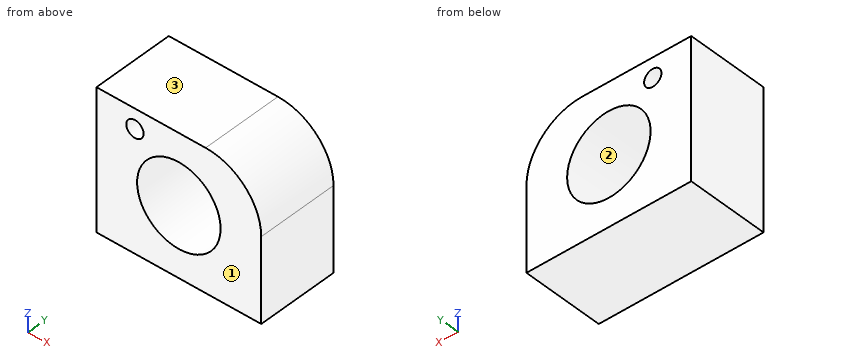
```python
from build123d import *

# Parameters (mm, degrees)
F0_W     = 88.888892
F0_H     = 75.277782
F1_DEPTH = 44
F2_R     = 22.514909
F3_DEPTH = 44.001
F4_R     = 4.664541
F5_DEPTH = 44.001
F6_R     = 30


with BuildPart() as f1:
    # F0 (on Front) → F1 (new body)
    with BuildSketch(Plane.XZ):
        Rectangle(F0_W, F0_H)
    extrude(amount=F1_DEPTH)

    # F2 (on face) → F3 (cut, through all)
    with BuildSketch(Plane.XZ.offset(44)):
        Circle(F2_R)
    extrude(amount=-F3_DEPTH, mode=Mode.SUBTRACT)

    # F4 (on face) → F5 (cut, through all)
    with BuildSketch(Plane.XZ.offset(44)):
        with Locations((-23.689743, 27.031031)):
            Circle(F4_R)
    extrude(amount=-F5_DEPTH, mode=Mode.SUBTRACT)

    # F6
    f6_edges = [f1.edges().sort_by_distance(p)[0] for p in [
        (44.444446, -22, 37.638891),
    ]]
    fillet(f6_edges, radius=F6_R)


solid = f1.part
```
Source: CAD feature listing. Evaluate the final solid. Frame: model axes, mm. Face numbers are marked on the shaded views. Coordinates: 2 decimals unless noted, no trailing zeros. Order: outer loops, then holes, each group sorted by start corner. A loop starts at its lowest first (then second) coordinate and runs counter-clockwise, first axis right, second up. Notation, with made-up numbers: M 86,-21.75 L 94,-21.75 A30 cw 94,3.25 Z; hole C 81,17.5 d1. An arc over 180 degrees is marked long. Write each question's results on one line, items separated by ' | '. Start each with the question number.
1) Section query A-A (z = 0). Return the cut outline in (x, y), plus the area to 3 significant figures.
2) Line query: line 1 (Z direction, x = 0, y = -21.5); line 2 (Z direction, x = -25, y = -11); line 3 (X direction, y = -38.5, z = -6). Output: solid intervals per line, ascending. Write a range as from..to.
3) Section query C-C (y = -25). Return the cut outline in (x, z), plus the area to 3 significant figures.
4) Draft query along Z for the marked faces 1, 2 and 3. Return one class per face: released by +Z, released by -Z, zero draft, split by the parting line, or undercut.
5) Contact query for a flat-ended pin moving along its axis: pin 1 Ø4 at (x, z) = (-1, 20) entering from -Y. Output: stop coordinate, or through.
6) Section query B-B (x = 0). Return the cut outline in (y, z), plus the area to 3 significant figures.
Answers:
1) outline: M -44.44,-44 L -22.51,-44 L -22.51,0 L -44.44,0 Z; M 22.51,-44 L 44.44,-44 L 44.44,0 L 22.51,0 Z | area: 1,930 mm^2
2) line 1: z = -37.64..-22.51, 22.51..37.64 | line 2: z = -37.64..22.55, 31.51..37.64 | line 3: x = -44.44..-21.7, 21.7..44.44
3) outline: M -44.44,-37.64 L 44.44,-37.64 L 44.44,7.64 A30 ccw 14.44,37.64 L -44.44,37.64 Z; hole C -23.69,27.03 d9.33; hole C 0,0 d45.03 | area: 4,840 mm^2
4) face 1: zero draft | face 2: undercut | face 3: released by +Z
5) pin 1: passes through
6) outline: M -44,-37.64 L 0,-37.64 L 0,-22.51 L -44,-22.51 Z; M -44,22.51 L 0,22.51 L 0,37.64 L -44,37.64 Z | area: 1,330 mm^2
